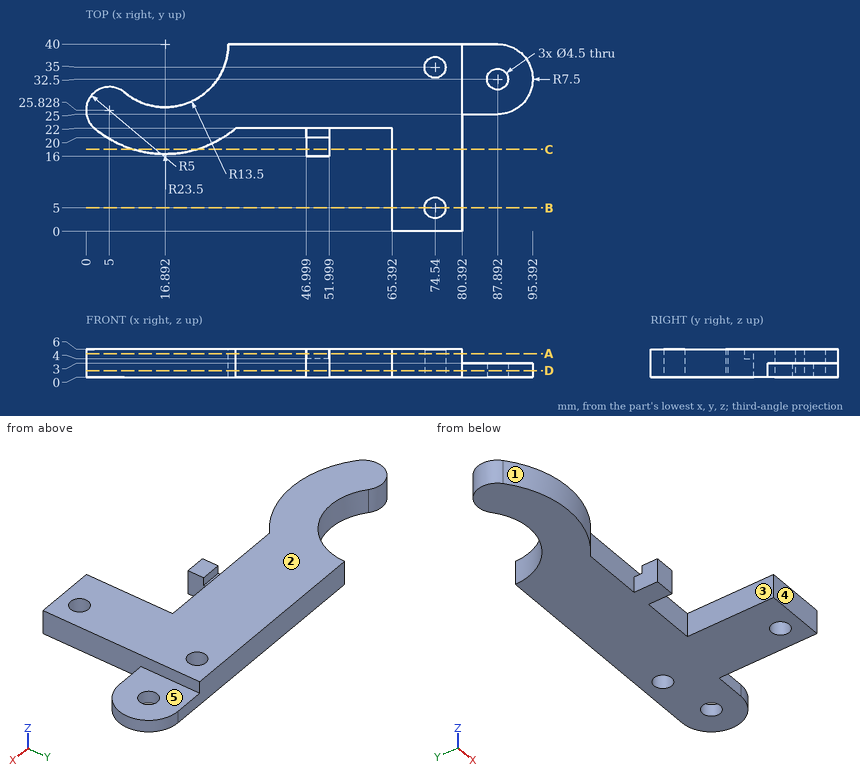
Verification items for this drawing (mm, ordinates from the low corner). A direction names the side the tool comes from. Coordinates: 2 decimals unless noted, no trailing zeros. Loops run counter-clockwise (first coordinate to the right, second up) from the corner with the lowest first, then second, coordinate; pieces in that order, holes last.
Item 1: Go/stop test with flat-tipped pins: pin 1 Ø2 at (x, z) = (80.5, 3.5) entering from -Y; pin 2 Ø3 at (y, z) = (20, 3.5) entering from -X; pin 3 Ø3 at (y, z) = (19.5, 3.5) entering from +X; pin 4 Ø0.6 at (x, y) = (48.5, 21) entering from +Z. Record where each tip stops, or that it passes through.
Item 2: Sectioned sample at C-C, the plane y = 17.5. Record the boundary of the cut face in (x, z).
Item 3: Thickness scan on line 1 (X direction, y = 5, z = 2.7); line 2 (X direction, y = 11.5, z = 0.45); line 3 (X direction, y = 6, z = 1.8) (1 decimal). Record the ranges inside material, lowest first.
Item 4: Release check for a two-part mould opening along X. For the marked faces 1 and 2 record: released by +X, released by -X, zero draft, split by the parting line, or undercut.
Item 5: Sectioned sample at B-B, the plane y = 5. Record the boundary of the cut face in (x, z), then the cut area to 3 significant figures.
Item 6: Access from +Z, -Z, +X, -X, +Y, -Y to the whole of each face (thin tool, end or side, straight path). Record for the marked faces 3, 4 and 5.
Item 7: Sectioned sample at A-A, the plane z = 5.1. Record the boundary of the cut face in (x, y), then the cut area to 3 significant figures.
Item 8: Sectioned sample at D-D, the plane z = 1.45. Record the boundary of the cut face in (x, y).
Check result:
1. pin 1: stops at y = 0
1. pin 2: stops at x = 2.4
1. pin 3: stops at x = 80.39
1. pin 4: stops at z = 4
2. outline: (10.11, 0) - (23.67, 0) - (23.67, 6) - (10.11, 6) - close; (47, 0) - (52, 0) - (52, 6) - (47, 6) - close; (65.39, 0) - (80.39, 0) - (80.39, 6) - (65.39, 6) - close
3. line 1: x = 65.39 to 72.29, 76.79 to 80.39
3. line 2: x = 65.39 to 80.39
3. line 3: x = 65.4 to 72.5, 76.6 to 80.4
4. face 1: undercut
4. face 2: zero draft
5. outline: (65.39, 0) - (72.29, 0) - (72.29, 6) - (65.39, 6) - close; (76.79, 0) - (80.39, 0) - (80.39, 6) - (76.79, 6) - close
5. area: 63.0 mm2
6. face 3: +Z, -Z, -Y
6. face 4: +Z, -Z, +X, -X, -Y
6. face 5: +Z, +X, +Y, -Y
7. outline: (1.79, 22) arc R23.5 ccw to (32, 22) - (65.39, 22) - (65.39, 0) - (80.39, 0) - (80.39, 40) - (30.39, 40) arc R13.5 cw to (8.21, 29.66) arc R5 ccw to start; (47, 16) - (52, 16) - (52, 20) - (47, 20) - close; hole circle Ø4.5 at (74.54, 5); hole circle Ø4.5 at (74.54, 35)
7. area: 1,540 mm2
8. outline: (1.79, 22) arc R23.5 ccw to (32, 22) - (47, 22) - (47, 16) - (52, 16) - (52, 22) - (65.39, 22) - (65.39, 0) - (80.39, 0) - (80.39, 25) - (87.89, 25) arc R7.5 ccw to (87.89, 40) - (30.39, 40) arc R13.5 cw to (8.21, 29.66) arc R5 ccw to start; hole circle Ø4.5 at (74.54, 5); hole circle Ø4.5 at (74.54, 35); hole circle Ø4.5 at (87.89, 32.5)
